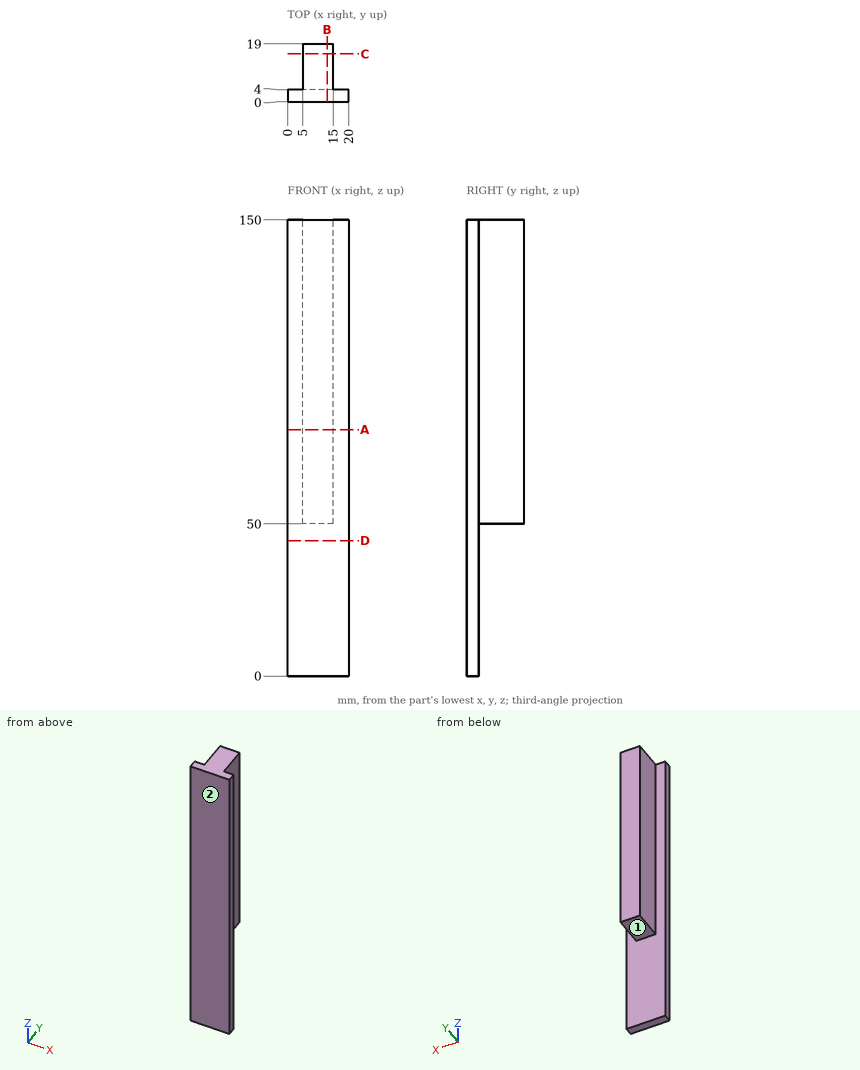
Study the drawing (mm; zero at the part's minimum x, y, z) and answer. A direction names the side the tool comes from. Coordinates: 2 decimals unless noted, no trailing zeros. Write each loop counter-clockwise with the first axis right and the second up, starting at its lowest first coordinate (ties: lowest second). Pieces come first, ordered by that corner, then holes. Notation, with made-up numbers: M -10.75,-33 L 15.25,-33 A22 cw 15.25,-3 Z; hole C 2.25,45.25 d11. An arc over 180 degrees is marked long. Use a Markdown table: item, result. Add a question column.
1. Given P1, Ø8, axis at y = 4, z = 113.5, coming from the -X side; P2, Ø3, axis at y = 16.5, z = 102.5, coming from the +X side; P3, Ø3, axis at x = 11, y = 14.5, coming from the -Z side, each flat-ended and moving along its own axis, determine where each tip first touches the part or whether it passes through.
2. Section B-B (x = 13) is taken. Give the vertices of the cut face in (y, z), plus the area to 3 significant figures.
3. Section C-C (y = 15.75) is taken. Give the vertices of the cut face in (x, z).
4. Which of the six approach directions +Z, -Z, +X, -X, +Y, -Y give full straight-line access (tool end or side, diameter ignored) to the marked faces 1 and 2?
5. Section A-A (z = 81) is taken. Give the vertices of the cut face in (x, y).
6. Section D-D (z = 44.5) is taken. Give the vertices of the cut face in (x, y), plus the area to 3 significant figures.
7. Straight lines are drawn through the part: line 1 along Z through (x, y) = (13, 9.25); line 2 along Y through (x, z) = (2.5, 31.5); line 3 along X through (y, z) = (7.75, 71). For each, find the intervals that lie inside material, in ascending order. Write a range as [from, to].
Data:
| question | item | result |
|---|---|---|
| 1 | P1 | stops at x = 0 |
| 1 | P2 | stops at x = 15 |
| 1 | P3 | stops at z = 50 |
| 2 | outline | M 0,0 L 4,0 L 4,50 L 19,50 L 19,150 L 0,150 Z |
| 2 | area | 2,100 mm2 |
| 3 | outline | M 5,50 L 15,50 L 15,150 L 5,150 Z |
| 4 | face 1 | -Z, +X, -X, +Y |
| 4 | face 2 | +Z, -Z, +X, -X, -Y |
| 5 | outline | M 0,0 L 20,0 L 20,4 L 15,4 L 15,19 L 5,19 L 5,4 L 0,4 Z |
| 6 | outline | M 0,0 L 20,0 L 20,4 L 0,4 Z |
| 6 | area | 80.0 mm2 |
| 7 | line 1 | z = [50, 150] |
| 7 | line 2 | y = [0, 4] |
| 7 | line 3 | x = [5, 15] |
